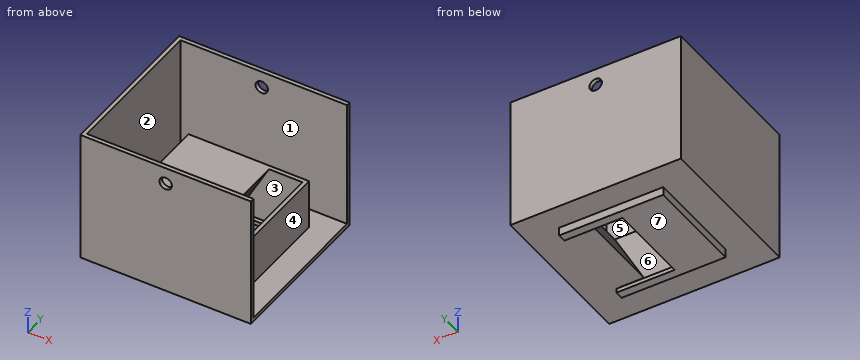
```python
from build123d import *

# Parameters (mm, degrees)
F0_W      = 130.175
F0_H      = 120.65
F1_DEPTH  = 101.6
F2_T      = -3.175
F3_W      = 85.725
F3_H      = 69.85
F4_DEPTH  = 25.4
F5_W      = 92.075
F5_H      = 76.2
F5_W_2    = 85.725
F5_H_2    = 69.85
F6_DEPTH  = 38.1
F7_W      = 79.375
F7_H      = 3.175
F8_DEPTH  = 6.35
F9_W      = 79.375
F9_H      = 3.175
F10_DEPTH = 6.35
F11_W     = 79.375
F11_H     = 3.175
F12_DEPTH = 3.175
F13_W     = 79.375
F13_H     = 3.175
F14_DEPTH = 3.175
F15_W     = 114.3
F15_H     = 95.25
F16_DEPTH = 6.35
F17_W     = 114.3
F17_H     = 3.175
F18_DEPTH = 16.764
F20_DEPTH = 69.85
F22_DEPTH = 69.85
F23_R     = 4.7625
F24_DEPTH = 148.082
F25_W     = 3.175
F25_H     = 3.175
F26_DEPTH = 69.85
F27_DEPTH = 3.175
F28_W     = 63.5
F28_H     = 3.175
F29_DEPTH = 31.75


with BuildPart() as f1:
    # F0 (on Top) → F1 (new body)
    with BuildSketch(Plane.XY):
        with Locations((244.3640923992, 60.325)):
            Rectangle(F0_W, F0_H)
    extrude(amount=F1_DEPTH)

    # F2
    f2_openings = [f1.faces().sort_by_distance(p)[0] for p in [
        (244.364092, 60.325, 101.6),
    ]]
    offset(amount=F2_T, openings=f2_openings)

    # F3 (on face) → F4 (cut)
    with BuildSketch(Plane.XY.offset(3.175)):
        with Locations((244.3640923992, 63.5)):
            Rectangle(F3_W, F3_H)
    extrude(amount=-F4_DEPTH, mode=Mode.SUBTRACT)

    # F5 (on face) → F6 (join)
    with BuildSketch(Plane.XY.offset(3.175)):
        with Locations((244.3640923992, 63.5)):
            Rectangle(F5_W, F5_H)
        with Locations((244.3640923992, 63.5)):
            Rectangle(F5_W_2, F5_H_2, mode=Mode.SUBTRACT)
    extrude(amount=F6_DEPTH)

    # F7 (on face) → F8 (join)
    with BuildSketch(Plane(origin=(0, 0, 0), x_dir=(1, 0, 0), z_dir=(0, 0, -1))):
        with Locations((244.3640923992, -26.9875)):
            Rectangle(F7_W, F7_H)
    extrude(amount=F8_DEPTH)

    # F9 (on face) → F10 (join)
    with BuildSketch(Plane(origin=(0, 0, 0), x_dir=(1, 0, 0), z_dir=(0, 0, -1))):
        with Locations((244.3640923992, -100.0125)):
            Rectangle(F9_W, F9_H)
    extrude(amount=F10_DEPTH)

    # F11 (on face) → F12 (join)
    with BuildSketch(Plane.XZ.offset(-98.425)):
        with Locations((244.3640923992, -4.7625)):
            Rectangle(F11_W, F11_H)
    extrude(amount=F12_DEPTH)

    # F13 (on face) → F14 (join)
    with BuildSketch(Plane(origin=(0, 28.575, 0), x_dir=(-1, 0, 0), z_dir=(0, 1, 0))):
        with Locations((-244.3640923992, -4.7625)):
            Rectangle(F13_W, F13_H)
    extrude(amount=F14_DEPTH)

    # F15 (on face) → F16 (cut)
    with BuildSketch(Plane.YZ.offset(309.4515923992)):
        with Locations((60.325, 50.8)):
            Rectangle(F15_W, F15_H)
    extrude(amount=-F16_DEPTH, mode=Mode.SUBTRACT)

    # F17 (on face) → F18 (cut)
    with BuildSketch(Plane.YZ.offset(309.4515923992)):
        with Locations((60.325, 100.0125)):
            Rectangle(F17_W, F17_H)
    extrude(amount=-F18_DEPTH, mode=Mode.SUBTRACT)

    # F19 (on face) → F20 (join)
    with BuildSketch(Plane.XZ.offset(-98.425)):
        Polygon((265.0015923992, 0), (284.0515923992, 0), (287.2265923992, 0), (287.2265923992, 41.275), align=None)
    extrude(amount=F20_DEPTH)

    # F21 (on face) → F22 (join)
    with BuildSketch(Plane.XZ.offset(-98.425)):
        Polygon((201.5015923992, 0), (204.6765923992, 0), (239.6015923992, 0), (261.8265923992, 41.275), (201.5015923992, 41.275), align=None)
    extrude(amount=F22_DEPTH)

    # F23 (on face) → F24 (cut)
    with BuildSketch(Plane.XZ):
        with Locations((244.3640923992, 88.9)):
            Circle(F23_R)
    extrude(amount=-F24_DEPTH, mode=Mode.SUBTRACT)

    # F25 (on face) → F26 (join)
    with BuildSketch(Plane(origin=(0, 28.575, 0), x_dir=(-1, 0, 0), z_dir=(0, 1, 0))):
        with Locations((-206.2640923992, -1.5875)):
            Rectangle(F25_W, F25_H)
    extrude(amount=F26_DEPTH)

    # F27 (add): a face of the model
    f27_faces = [f1.faces().sort_by_distance(p)[0] for p in [
        (206.2640923992, 63.5, -3.175),
    ]]
    extrude(f27_faces, amount=F27_DEPTH)

    # F28 (on face) → F29 (join)
    with BuildSketch(Plane.YZ.offset(207.8515923992)):
        with Locations((63.5, -4.7625)):
            Rectangle(F28_W, F28_H)
    extrude(amount=F29_DEPTH)


solid = f1.part
```
CAD build for the part. Positions are in the model's coordinates, mm. Face numbers are marked on the shaded views. A direction names the side the tool comes from. Round coordinates to 2 decimals unless told otherwise and drop trailing zeros. Write each loop counter-clockwise with the first axis right and the second up, starting at its lowest first coordinate (ties: lowest second). Pieces come first, ordered by that corner, then holes. Notation, with made-up numbers: (58.25, 76) -> (97.25, 76) arc R21 cw to (97.25, 102) -> close; hole circle Ø9 at (45.5, 85). An arc over 180 degrees is marked (long way). Answer in a Markdown table with one row per item. Add a question column.
Item 1: Mould opens along X. For the marked faces 1, 2, 3 and 4 say: pulls with the +X half, pulls with the -X half, needs draft (parallel to the pull), parting line crosses it, or undercut.
Item 2: Drop flat-ended pins along their axis: pin 1 Ø1.6 at (x, z) = (271.5, -4.5) entering from +Y; pin 2 Ø5 at (x, y) = (224, 19) entering from +Z (3 decimals); pin 3 Ø21 at (x, y) = (255.5, 81) entering from +Z (3 decimals); pin 4 Ø10 at (x, z) = (276.5, 22.5) entering from -Y. Give the stop position or say it passes through.
Item 3: Saw through at A-A, the plane y = 37. Write the cut outline in (x, z) (3 decimals), then the cut area to 3 significant figures.
Item 4: Drill centre lines: line 1 (Y direction, x = 276, z = 17) (3 decimals); line 2 (Y direction, x = 272.5, z = 39) (3 decimals); line 3 (Y direction, x = 271, z = 72) (3 decimals). Where is each one in solid material? Low to high. Write a range as from..to.
Item 5: Saw through at C-C, the plane x = 230. Write the cut outline in (y, z) (3 decimals), then the cut area to 3 significant figures.
Item 6: Saw through at D-D, the plane z = 28.5. Write the cut outline in (x, y) (3 decimals).
Item 7: Saw through at B-B, the plane z = 88.9. Write the cut outline in (x, y) (3 decimals), then the cut area to 3 significant figures.
Item 8: Which spindle directions (+Z, -Z, +X, -X, +Y, -Y) get a long thin tool onto all of the face, cutting with end or side? Do the marked faces 5, 6 and 7. Say none if no direction does.
Findings below:
| question | item | result |
|---|---|---|
| 1 | face 1 | needs draft |
| 1 | face 2 | undercut |
| 1 | face 3 | undercut |
| 1 | face 4 | pulls with the +X half |
| 2 | pin 1 | stops at y = 101.6 |
| 2 | pin 2 | stops at z = 3.175 |
| 2 | pin 3 | stops at z = 41.275 |
| 2 | pin 4 | stops at y = 0 |
| 3 | outline | (179.277, 0) -> (204.677, 0) -> (204.677, -6.35) -> (239.602, -6.35) -> (239.602, -3.175) -> (207.852, -3.175) -> (207.852, 0) -> (239.602, 0) -> (261.827, 41.275) -> (198.327, 41.275) -> (198.327, 3.175) -> (182.452, 3.175) -> (182.452, 101.6) -> (179.277, 101.6) -> close; (265.002, 0) -> (309.452, 0) -> (309.452, 3.175) -> (290.402, 3.175) -> (290.402, 41.275) -> (287.227, 41.275) -> close |
| 3 | area | 3,310 mm^2 |
| 4 | line 1 | y = 0..3.175, 25.4..101.6, 117.475..120.65 |
| 4 | line 2 | y = 0..3.175, 25.4..28.575, 98.425..101.6, 117.475..120.65 |
| 4 | line 3 | y = 0..3.175, 117.475..120.65 |
| 5 | outline | (0, 0) -> (25.4, 0) -> (25.4, -6.35) -> (101.6, -6.35) -> (101.6, 0) -> (120.65, 0) -> (120.65, 101.6) -> (117.475, 101.6) -> (117.475, 3.175) -> (101.6, 3.175) -> (101.6, 41.275) -> (25.4, 41.275) -> (25.4, 3.175) -> (3.175, 3.175) -> (3.175, 101.6) -> (0, 101.6) -> close; hole (28.575, -3.175) -> (98.425, -3.175) -> (98.425, 0) -> (28.575, 0) -> close |
| 5 | area | 4,170 mm^2 |
| 6 | outline | (179.277, 0) -> (309.452, 0) -> (309.452, 3.175) -> (182.452, 3.175) -> (182.452, 117.475) -> (309.452, 117.475) -> (309.452, 120.65) -> (179.277, 120.65) -> close; (198.327, 25.4) -> (290.402, 25.4) -> (290.402, 101.6) -> (198.327, 101.6) -> close; hole (254.948, 28.575) -> (280.348, 28.575) -> (280.348, 98.425) -> (254.948, 98.425) -> close |
| 7 | outline | (179.277, 0) -> (239.602, 0) -> (239.602, 3.175) -> (182.452, 3.175) -> (182.452, 117.475) -> (239.602, 117.475) -> (239.602, 120.65) -> (179.277, 120.65) -> close; (249.127, 0) -> (309.452, 0) -> (309.452, 3.175) -> (249.127, 3.175) -> close; (249.127, 117.475) -> (309.452, 117.475) -> (309.452, 120.65) -> (249.127, 120.65) -> close |
| 7 | area | 1,130 mm^2 |
| 8 | face 5 | +Z, +X |
| 8 | face 6 | none |
| 8 | face 7 | -Z, +X, -X, +Y, -Y |
